Autodesk Inventor part; units mm, degrees
ref_plane "YZ Plane" through (0, 0, 0) normal (1, 0, 0) x (0, 1, 0)
ref_plane "XZ Plane" through (0, 0, 0) normal (0, 1, 0) x (-1, 0, 0)
ref_plane "XY Plane" through (0, 0, 0) normal (0, 0, 1) x (1, 0, 0)
sketch "草圖2" plane through (0, 0, 0) normal (0, 0, 1) x (1, 0, 0)
  line L0 (0, 55) -> (0, 0)
  line L1 (0, 0) -> (22, 0)
  line L2 (22, 0) -> (22, 44)
  line L3 (22, 44) -> (154, 44)
  line L4 (154, 44) -> (154, 0)
  line L5 (154, 0) -> (176, 0)
  line L6 (176, 0) -> (176, 55)
  line L7 (176, 55) -> (0, 55)
  dimension "d11" = 22
  dimension "d12" = 11
  dimension "d14" = 176
  dimension "d17" = 44
extrude "擠出2" add sketch "草圖2" along normal mid plane 176
equation "\"d11\" = leg_length"
equation "\"d12\" = thickness"
equation "\"d14\" = width"
equation "\"d17\" = height"
equation "\"d15\" = length"
equation "\"width\" = 8 * ratio"
equation "\"height\" = 2 * ratio"
equation "\"length\" = width"
equation "\"leg_length\" = ratio"
equation "\"ratio\" = 2.2"
equation "\"thickness\" = 0.5 * ratio"
properties part number "bridge_rect_final"
Here's how the part is built. I have some questions about the finished solid (model axes, mm). A direction names the side the tool comes from. Round coordinates to 2 decimals unless told otherwise and drop trailing zeros. Order: outer loops, then holes, each group sorted by start corner. A loop starts at its lowest first (then second) coordinate and runs counter-clockwise, first axis right, second up. Notation, with made-up numbers: (-12, 29.25) -> (2, 29.25) arc R10 ccw to (2, 46.25) -> close; hole circle Ø1 at (72.5, -16.5). An arc over 180 degrees is marked (long way). Return JSON: item names as keys, results as strings.
Q1. I need wall thicknesses on line 1 along X through (y, z) = (20, 2); line 2 along Y through (x, z) = (118.5, -9). Which ranges of each line are inside material? Lowest first, please. Write a range as from..to.
Filled sheet:
{"line 1": "x = 0..22, 154..176", "line 2": "y = 44..55"}
Q2. For pin 1 Ø12 at (y, z) = (42, 59.5) entering from -X; pin 2 Ø1 at (x, z) = (65.5, 58.5) entering from -Y, each with a flat end and sliding along its axis, tell me the tip position at first contact or that it passes through.
Filled sheet:
{"pin 1": "stops at x = 0", "pin 2": "stops at y = 44"}
Q3. Which directions (+Z, -Z, +X, -X, +Y, -Y) give clear straight access to the entire face, cutting with the end or side of a thin tool? Please do faces 1 (the flat face through (154, 22, -1)), 2 (the flat face through (87, 46, 88)).
Filled sheet:
{"face 1": "+Z, -Z, -Y", "face 2": "+Z, +X, -X, +Y, -Y"}
Q4. If we section it at C-C on x = 128.5: List the corners of the cut face in (y, z) for me.
Filled sheet:
{"outline": "(44, -88) -> (55, -88) -> (55, 88) -> (44, 88) -> close"}
Q5. If we section it at A-A on y = 27.5: List the corners of the cut face in (x, z) for me.
Filled sheet:
{"outline": "(0, -88) -> (22, -88) -> (22, 88) -> (0, 88) -> close; (154, -88) -> (176, -88) -> (176, 88) -> (154, 88) -> close"}
Q6. If we section it at B-B on z = -14: List the corners of the cut face in (x, y) for me, plus the area to 3 significant figures.
Filled sheet:
{"outline": "(0, 0) -> (22, 0) -> (22, 44) -> (154, 44) -> (154, 0) -> (176, 0) -> (176, 55) -> (0, 55) -> close", "area": "3,870 mm^2"}
Q7. If we mould it in two halves opening along X, with no side actions, what happens to faces 3 (the flat face through (22, 22, -1)), 4 (the flat face through (0, 28, -1)), 5 (the flat face through (87, 44, -1)), 6 (the flat face through (89, 55, -1))? For each: released by +X, released by -X, zero draft, split by the parting line, or undercut.
Filled sheet:
{"face 3": "undercut", "face 4": "released by -X", "face 5": "undercut", "face 6": "zero draft"}
